from build123d import *

# Parameters (mm, degrees)
SKETCH1_R               = 4.4
BOSS_EXTRUDE1_DEPTH     = 10
SKETCH1_2_R             = 4.4
BOSS_EXTRUDE2_DEPTH     = 2
SKETCH3_W               = 30
SKETCH3_H               = 12
BOSS_EXTRUDE4_DEPTH     = 7.2
CUT_EXTRUDE2_START      = -12.2
SKETCH2_R               = 1.65
CUT_EXTRUDE2_DEPTH      = 8
SKETCH5_W               = 30
SKETCH5_H               = 3.15
CUT_EXTRUDE3_DEPTH      = 23.756098084
CUT_EXTRUDE3_DEPTH_BACK = 3.15
SKETCH6_W               = 14
SKETCH6_H               = 3.15
CUT_EXTRUDE4_DEPTH      = 23.756098084
CUT_EXTRUDE4_DEPTH_BACK = 23.756098084


with BuildPart() as part:
    # Sketch1 → Boss-Extrude1 (new body)
    with BuildSketch(Plane.XY):
        with BuildLine():
            Line((-15, -5), (15, -5))
            ThreePointArc((15, -5), (10.104984149, -1.836764635), (6.785093744, 2.953388374))
            ThreePointArc((6.785093744, 2.953388374), (0, 7.4), (-6.785093744, 2.953388374))
            ThreePointArc((-6.785093744, 2.953388374), (-10.104984149, -1.836764635), (-15, -5))
        make_face()
        Circle(SKETCH1_R, mode=Mode.SUBTRACT)
    extrude(amount=BOSS_EXTRUDE1_DEPTH)

    # Sketch1<2> → Boss-Extrude2 (add)
    with BuildSketch(Plane.XY):
        with BuildLine():
            ThreePointArc((-6.785093744, 2.953388374), (0, 7.4), (6.785093744, 2.953388374))
            ThreePointArc((6.785093744, 2.953388374), (10.104984149, -1.836764635), (15, -5))
            Line((15, -5), (-15, -5))
            ThreePointArc((-15, -5), (-10.104984149, -1.836764635), (-6.785093744, 2.953388374))
        make_face()
        Circle(SKETCH1_2_R, mode=Mode.SUBTRACT)
        Circle(SKETCH1_2_R)
    extrude(amount=-BOSS_EXTRUDE2_DEPTH)

    # Sketch3 → Boss-Extrude4 (add)
    with BuildSketch(Plane.XZ.offset(5)):
        with Locations((0, 4)):
            Rectangle(SKETCH3_W, SKETCH3_H)
    extrude(amount=BOSS_EXTRUDE4_DEPTH)

    # Sketch2 → Cut-Extrude2 (cut)
    with BuildSketch(Plane(origin=(0, 0, 0), x_dir=(1, 0, 0), z_dir=(0, 1, 0)).offset(CUT_EXTRUDE2_START)):
        with Locations(Location((-11.5, -4, 0), (0, 0, 90))):
            Circle(SKETCH2_R)
        with Locations(Location((11.5, -4, 0), (0, 0, 90))):
            Circle(SKETCH2_R)
    extrude(amount=CUT_EXTRUDE2_DEPTH, mode=Mode.SUBTRACT)

    # Sketch5 → Cut-Extrude3 (cut, two sides)
    with BuildSketch(Plane(origin=(0, 0, -2), x_dir=(-1, 0, 0), z_dir=(0, 0, -1))) as cut_extrude3_sk:
        with Locations((0, -10.625)):
            Rectangle(SKETCH5_W, SKETCH5_H)
    extrude(amount=CUT_EXTRUDE3_DEPTH, mode=Mode.SUBTRACT)
    extrude(cut_extrude3_sk.sketch, amount=-CUT_EXTRUDE3_DEPTH_BACK, mode=Mode.SUBTRACT)

    # Sketch6 → Cut-Extrude4 (cut, two sides)
    with BuildSketch(Plane.XY.offset(10)) as cut_extrude4_sk:
        with Locations((0, -10.625)):
            Rectangle(SKETCH6_W, SKETCH6_H)
    extrude(amount=CUT_EXTRUDE4_DEPTH, mode=Mode.SUBTRACT)
    extrude(cut_extrude4_sk.sketch, amount=-CUT_EXTRUDE4_DEPTH_BACK, mode=Mode.SUBTRACT)


solid = part.part
Design review of the part built by this model. Coordinates are the model's own, in mm. A direction names the side the tool comes from. Coordinates: 2 decimals unless noted, no trailing zeros. Order: outer loops, then holes, each group sorted by start corner. A loop starts at its lowest first (then second) coordinate and runs counter-clockwise, first axis right, second up. Notation, with made-up numbers: (69.5, 56.5) -> (106.5, 56.5) arc R33 cw to (106.5, 89.5) -> close; hole circle Ø2 at (-16.75, 81.25). An arc over 180 degrees is marked (long way). Use one line per item in the form item = value. Start each with the question number.
(1) Add section C-C on y = 0.75. State the section outline as (x, z) points, plus the area to 3 significant figures.
(2) For faces 1 (the flat face through (11, -4.2, 4)), 2 (the flat face through (-11, -11, 1.15)), 3 (the flat face through (7, -11, 6)), list the 3-axis set-ups (+Z, -Z, +X, -X, +Y, -Y) from which the entire face can be reached by the end or side of a thin tool; tool diameter is ignored.
(3) The part is to be moulded in two halves that separate along Y. For faces 4 (the flat face through (-11, -12.2, 6)), 5 (the cylindrical face through (-10.16, -1.89, 4.08)), 6 (the flat face through (11, -11, 1.15)), 7 (the flat face through (0, 0, 0)), say which applies: +Y half, -Y half, draft (parallel to the pull), parting line (faces both ways), or undercut.
(4) Add section D-D on z = 4. State the section outline as (x, y) points, plus the area to 3 significant figures.
(5) Insertion check: pin 1 (1 mm diameter, centred on y = -0.5, z = 8.5, fed in from -X); pin 2 (2.5 mm diameter, centred on x = -1.5, y = -1.5, fed in from +Z); pin 3 (1.6 mm diameter, centred on x = 9, y = -10.5, fed in from -Z). Each pin has a flat end and moves straight along its axis. Give the tip position at first contact, or say it passes through.
(6) Add section B-B on x = 0. State the section outline as (y, z) points.
(7) Add section A-A on z = 9. State the section outline as (x, y) points, plus the area to 3 significant figures.
(8) For probe 1 along X at (y, z) = (-7, 4); probe 2 along X at (y, z) = (-10.25, 4); probe 3 along Z at (x, y) = (11.5, -8.5), list the stretches that pass through material, from the lowest coordinate up.
Answer block:
q1.outline = (-7.97, -2) -> (7.97, -2) -> (7.97, 10) -> (4.34, 10) -> (4.34, 0) -> (-4.34, 0) -> (-4.34, 10) -> (-7.97, 10) -> close
q1.area = 105 mm²
q2.face_1 = -Y
q2.face_2 = -Z, +X, -X, -Y
q2.face_3 = +Z, -Z, -Y
q3.face_4 = -Y half
q3.face_5 = +Y half
q3.face_6 = draft
q3.face_7 = undercut
q4.outline = (-15, -12.2) -> (-13.15, -12.2) -> (-13.15, -4.2) -> (-9.85, -4.2) -> (-9.85, -12.2) -> (-7, -12.2) -> (-7, -9.05) -> (7, -9.05) -> (7, -12.2) -> (9.85, -12.2) -> (9.85, -4.2) -> (13.15, -4.2) -> (13.15, -12.2) -> (15, -12.2) -> (15, -5) arc R15 cw to (6.79, 2.95) arc R7.4 ccw to (-6.79, 2.95) arc R15 cw to (-15, -5) -> close; hole circle Ø8.8 at (0, 0)
q4.area = 258 mm²
q5.pin_1 = -9.3
q5.pin_2 = 0
q5.pin_3 = 1.15
q6.outline = (-9.05, -2) -> (7.4, -2) -> (7.4, 10) -> (4.4, 10) -> (4.4, 0) -> (-4.4, 0) -> (-4.4, 10) -> (-9.05, 10) -> close
q7.outline = (-15, -12.2) -> (-7, -12.2) -> (-7, -9.05) -> (7, -9.05) -> (7, -12.2) -> (15, -12.2) -> (15, -5) arc R15 cw to (6.79, 2.95) arc R7.4 ccw to (-6.79, 2.95) arc R15 cw to (-15, -5) -> close; hole circle Ø8.8 at (0, 0)
q7.area = 310 mm²
q8.probe_1 = -15 to -13.15, -9.85 to 9.85, 13.15 to 15
q8.probe_2 = -15 to -13.15, -9.85 to -7, 7 to 9.85, 13.15 to 15
q8.probe_3 = -2 to 2.35, 5.65 to 10
